Geometry check sheet. Reference: the model listing, model coordinates, mm. Face numbers are marked on the shaded views. Give positions to 0.01 mm unless a question says otherwise; leave off trailing zeros. Write each loop counter-clockwise with the first axis right and the second up, starting at its lowest first coordinate (ties: lowest second). Pieces come first, ordered by that corner, then holes. Notation, with made-up numbers: (10.25, 4.25) - (66.25, 4.25) arc R27 cw to (66.25, 31.25) - close; hole circle Ø6 at (86.25, -30.75). An arc over 180 degrees is marked (long way). Use a Markdown table: item, result.
```python
from build123d import *

# Parameters (mm, degrees)
SKETCH1_W           = 140
SKETCH1_H           = 250
BOSS_EXTRUDE1_DEPTH = 25
SKETCH2_W           = 128
SKETCH2_H           = 238
CUT_EXTRUDE1_DEPTH  = 23
SKETCH4_W           = 134
SKETCH4_H           = 244
CUT_EXTRUDE2_DEPTH  = 3


with BuildPart() as part:
    # Sketch1 → Boss-Extrude1 (new body)
    with BuildSketch(Plane(origin=(0, 0, 0), x_dir=(1, 0, 0), z_dir=(0, 1, 0))):
        Rectangle(SKETCH1_W, SKETCH1_H)
    extrude(amount=BOSS_EXTRUDE1_DEPTH)

    # Sketch2 → Cut-Extrude1 (cut)
    with BuildSketch(Plane(origin=(0, 25, 0), x_dir=(1, 0, 0), z_dir=(0, 1, 0))):
        Rectangle(SKETCH2_W, SKETCH2_H)
    extrude(amount=-CUT_EXTRUDE1_DEPTH, mode=Mode.SUBTRACT)

    # Sketch4 → Cut-Extrude2 (cut)
    with BuildSketch(Plane(origin=(0, 25, 0), x_dir=(1, 0, 0), z_dir=(0, 1, 0))):
        Rectangle(SKETCH4_W, SKETCH4_H)
    extrude(amount=-CUT_EXTRUDE2_DEPTH, mode=Mode.SUBTRACT)


solid = part.part
```
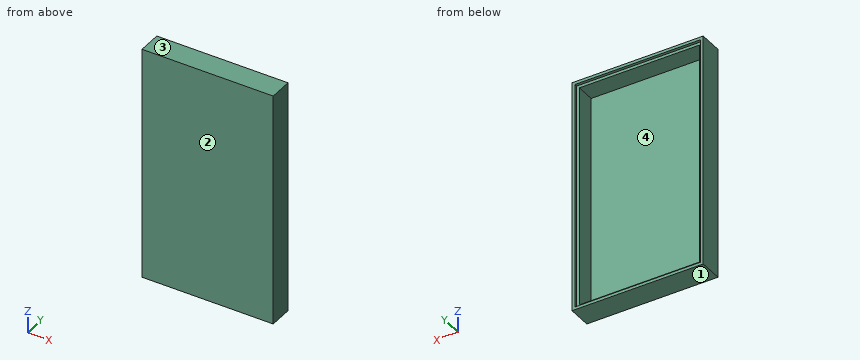
1) Mould release check, pull along Z, two halves, no side actions. Record for the marked faces 1, 2, 3 and 4: pulls with the +Z half, pulls with the -Z half, needs draft (parallel to the pull), parting line crosses it, or undercut.
Working result:
| item | result |
|---|---|
| face 1 | pulls with the -Z half |
| face 2 | needs draft |
| face 3 | pulls with the +Z half |
| face 4 | undercut |
2) Section check B-B on x = -47.5. Record the boundary of the cut face in (y, z).
Working result:
| item | result |
|---|---|
| outline | (0, -125) - (25, -125) - (25, -122) - (22, -122) - (22, -119) - (2, -119) - (2, 119) - (22, 119) - (22, 122) - (25, 122) - (25, 125) - (0, 125) - close |
3) Section check A-A on y = 6.25. Record the boundary of the cut face in (x, z), then the cut area to 3 significant figures.
Working result:
| item | result |
|---|---|
| outline | (-70, -125) - (70, -125) - (70, 125) - (-70, 125) - close; hole (-64, -119) - (64, -119) - (64, 119) - (-64, 119) - close |
| area | 4,540 mm² |
4) Material ranges on L1, parallel to Z at x = -10.5, y = 17.75; L2, parallel to X at y = 14.5, z = 34.5; L3, parallel to X at y = 23.5, z = 83.5, recorded low to high. Write a range as from..to.
Working result:
| item | result |
|---|---|
| L1 | z = -125..-119, 119..125 |
| L2 | x = -70..-64, 64..70 |
| L3 | x = -70..-67, 67..70 |
5) Section check C-C on z = 12.5. Record the boundary of the cut face in (x, y), then the cut area to 3 significant figures.
Working result:
| item | result |
|---|---|
| outline | (-70, 0) - (70, 0) - (70, 25) - (67, 25) - (67, 22) - (64, 22) - (64, 2) - (-64, 2) - (-64, 22) - (-67, 22) - (-67, 25) - (-70, 25) - close |
| area | 538 mm² |
6) Depth check by flat-ended pin: P1, Ø1.5, axis at x = 20, z = -96, coming from the +Y side. Enter the tip coordinate at first touch or a pass-through.
Working result:
| item | result |
|---|---|
| P1 | stops at y = 2 |
